Part model, mm, in its own coordinate system. A direction names the side the tool comes from. Give positions to 0.01 mm unless a question says otherwise; leave off trailing zeros. Order: outer loops, then holes, each group sorted by start corner. A loop starts at its lowest first (then second) coordinate and runs counter-clockwise, first axis right, second up.
1. Mould opens along X. For faces 5 (the flat face through (63.25, 37, 3)), 6 (the flat face through (-54, -40.25, 3)), 7 (the flat face through (31.2, 30.46, 2.96)) say: +X half, -X half, draft (parallel to the pull), parting line (faces both ways), or undercut.
2. Probe line 1 (Y direction, x = 0, z = 2.9); line 2 (X direction, y = 30.5, z = 0.45); line 3 (Y direction, x = 30, z = 0.95). List the from-to ranges inside material, lowest first.
3. Which spindle directions (+Z, -Z, +X, -X, +Y, -Y) get a long thin tool onto all of the face, cutting with end or side? Do faces 1 (the flat face through (-59.25, -35, 3)), 2 (the flat face through (-30.69, 30.12, 2.96)), 3 (the flat face through (-42.88, 19.022, 2.958)), 4 (the flat face through (0, 0, 1)). Say none if no direction does.
4. Slice it at C-C on x = -43. List the corners of the cut face in (y, z), and give its area (3 significant figures).
5. Slice it at A-A on y = 0. List the corners of the cut face in (x, z).
6. Drop flat-ended pins along their axis: pin 1 Ø1 at (y, z) = (-41, 3) entering from -X; pin 2 Ø3 at (y, z) = (-21.5, 2) entering from +X; pin 3 Ø1.5 at (y, z) = (-20, 3) entering from -X. Give the stop position or say it passes through.
from build123d import *

# Parameters (mm, degrees)
F0_R     = 17.5
F1_DEPTH = 6
F2_DEPTH = 1


with BuildPart() as f1:
    # F0 (on Top) → F1 (new body)
    with BuildSketch(Plane.XY):
        with BuildLine():
            Line((-59.25, -40.25), (-59.25, -42.25))
            Line((-59.25, -42.25), (-48.847482, -42.25))
            Line((-48.847482, -42.25), (-13.043494, -18.333501))
            ThreePointArc((-13.043494, -18.333501), (0, -22.5), (13.043494, -18.333501))
            Line((13.043494, -18.333501), (48.847482, -42.25))
            Line((48.847482, -42.25), (63.25, -42.25))
            Line((63.25, -42.25), (63.25, -32.629346))
            Line((63.25, -32.629346), (21.930829, -5.028793))
            ThreePointArc((21.930829, -5.028793), (22.5, 0), (21.930829, 5.028793))
            Line((21.930829, 5.028793), (63.25, 32.629346))
            Line((63.25, 32.629346), (63.25, 42.25))
            Line((63.25, 42.25), (48.847482, 42.25))
            Line((48.847482, 42.25), (13.043494, 18.333501))
            ThreePointArc((13.043494, 18.333501), (0, 22.5), (-13.043494, 18.333501))
            Line((-13.043494, 18.333501), (-48.847482, 42.25))
            Line((-48.847482, 42.25), (-63.25, 42.25))
            Line((-63.25, 42.25), (-63.25, 32.629346))
            Line((-63.25, 32.629346), (-21.930829, 5.028793))
            ThreePointArc((-21.930829, 5.028793), (-22.5, 0), (-21.930829, -5.028793))
            Line((-21.930829, -5.028793), (-63.25, -32.629346))
            Line((-63.25, -32.629346), (-63.25, -38.25))
            Line((-63.25, -38.25), (-61.25, -38.25))
            Line((-61.25, -38.25), (-61.25, -32.629346))
            Line((-61.25, -32.629346), (-59.25, -32.629346))
            Line((-59.25, -32.629346), (-59.25, -38.25))
            Line((-59.25, -38.25), (-48.847482, -38.25))
            Line((-48.847482, -38.25), (-48.847482, -40.25))
            Line((-48.847482, -40.25), (-59.25, -40.25))
        make_face()
        Circle(F0_R, mode=Mode.SUBTRACT)
    extrude(amount=F1_DEPTH)

    # F0 (on Top) → F2 (join)
    with BuildSketch(Plane.XY):
        Circle(F0_R)
    extrude(amount=F2_DEPTH)


solid = f1.part
Data:
1. face 5: +X half
1. face 6: draft
1. face 7: undercut
2. line 1: y = -22.5 to -17.5, 17.5 to 22.5
2. line 2: x = -60.06 to -31.26, 31.26 to 60.06
2. line 3: y = -29.66 to -10.42, 10.42 to 29.66
3. face 1: +Z, -Z, -Y
3. face 2: +Z, -Z, +Y
3. face 3: +Z, -Z, -X
3. face 4: +Z
4. outline: (-38.34, 0) - (-19.1, 0) - (-19.1, 6) - (-38.34, 6) - close; (19.1, 0) - (38.34, 0) - (38.34, 6) - (19.1, 6) - close
4. area: 231 mm2
5. outline: (-22.5, 0) - (22.5, 0) - (22.5, 6) - (17.5, 6) - (17.5, 1) - (-17.5, 1) - (-17.5, 6) - (-22.5, 6) - close
6. pin 1: stops at x = -59.25
6. pin 2: stops at x = 48.83
6. pin 3: stops at x = -45.47
